Geometry: see drawing. Coordinates: mm, zero at the bounding-box minimum. A direction names the side the tool comes from. Round coordinates to 2 decimals unless told otherwise and drop trailing zeros. Loops run counter-clockwise (first coordinate to the right, second up) from the corner with the lowest first, then second, coordinate; pieces in that order, holes last.
(1) Section C-C, the plane y = 5. Return the cut outline in (x, z).
(2) Set-up query: the marked faces 4, 5 and 6. Return all of +Z, -Z, +X, -X, +Y, -Y with unobstructed straight access to the full face (end or side cutting, diameter ignored); none if empty.
(3) Section B-B, the plane z = 7.5. Return the cut outline in (x, y), plus the area to 3 significant figures.
(4) Mould query, pull axis Y, two halves, no side actions, for the marked faces 1, 2 and 3. Classes: pulls with the +Y half, pulls with the -Y half, needs draft (parallel to the pull), parting line crosses it, or undercut.
(5) Section D-D, the plane y = 27.5. Return the cut outline in (x, z).
(6) Section A-A, the plane x = 6.5. Return the cut outline in (y, z).
(7) First-contact query: pin 1 Ø7 at (y, z) = (5.5, 8) entering from -X; pin 2 Ø2 at (x, z) = (5.5, 0.5) entering from -Y; pin 3 Ø7 at (y, z) = (3.5, 4.5) entering from +X. Flat tips, straight axial feed; report the tip coordinate or a pass-through.
(8) Material intervals for probe 1 along Y at (x, z) = (2, 8.5); probe 2 along Z at (x, y) = (9.75, 6.5); probe 3 along Y at (x, z) = (5.5, 11.5), sorted ascending.
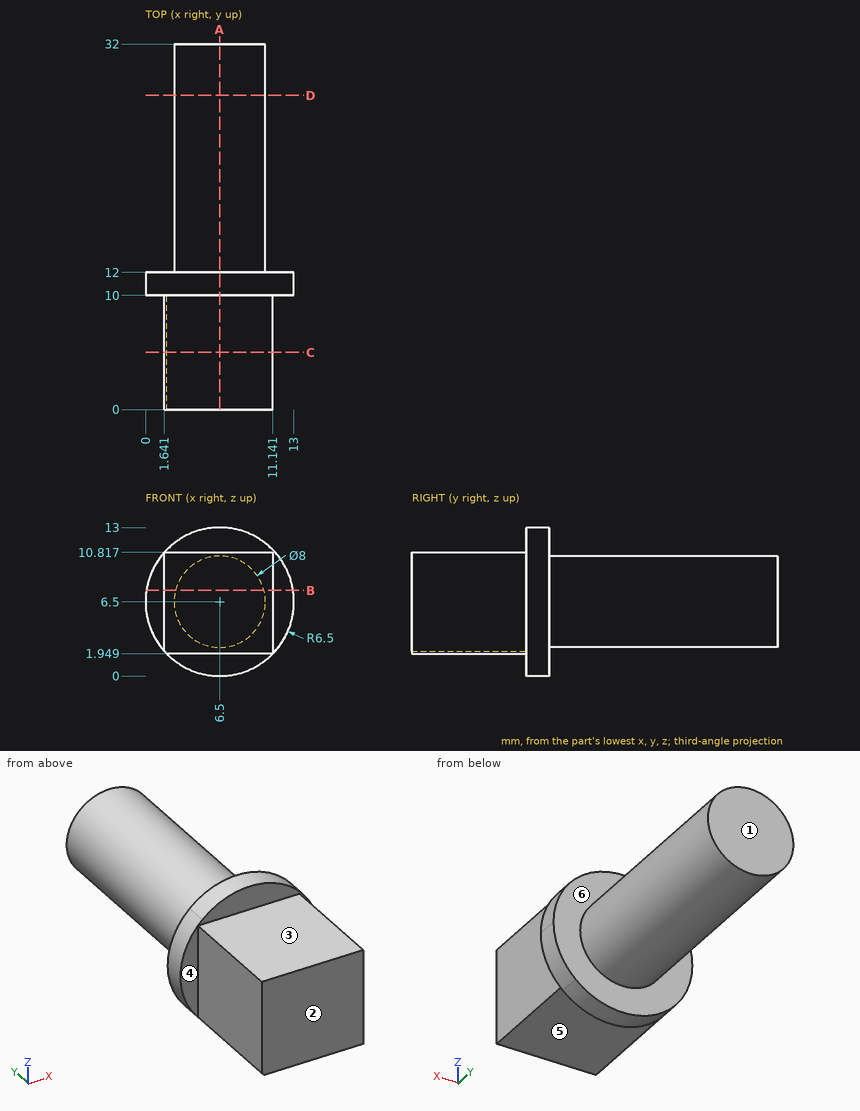
Output values:
1. outline: (1.64, 2.18) arc R6.5 ccw to (1.86, 1.95) - (11.14, 1.95) - (11.14, 10.82) - (1.64, 10.82) - close
2. face 4: +Z, -Z, -X, -Y
2. face 5: -Z, +X, -X, -Y
2. face 6: +Y
3. outline: (0.08, 10) - (1.64, 10) - (1.64, 0) - (11.14, 0) - (11.14, 10) - (12.92, 10) - (12.92, 12) - (10.37, 12) - (10.37, 32) - (2.63, 32) - (2.63, 12) - (0.08, 12) - close
3. area: 276 mm2
4. face 1: pulls with the +Y half
4. face 2: pulls with the -Y half
4. face 3: needs draft
5. outline: circle Ø8 at (6.5, 6.5)
6. outline: (0, 1.95) - (10, 1.95) - (10, 0) - (12, 0) - (12, 2.5) - (32, 2.5) - (32, 10.5) - (12, 10.5) - (12, 13) - (10, 13) - (10, 10.82) - (0, 10.82) - close
7. pin 1: stops at x = 1.64
7. pin 2: stops at y = 10
7. pin 3: stops at x = 11.14
8. probe 1: y = 0 to 12
8. probe 2: z = 1.95 to 10.82
8. probe 3: y = 10 to 12
